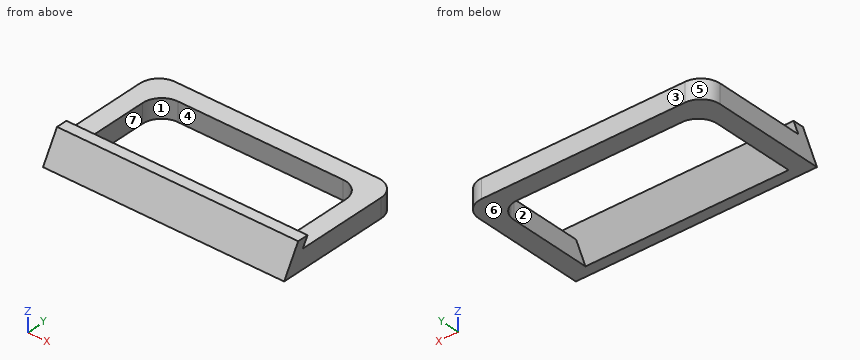
```python
from build123d import *

# Parameters (mm, degrees)
SALIENTE_EXTRUIR1_DEPTH = 10
SALIENTE_EXTRUIR2_DEPTH = 127


with BuildPart() as part:
    # Croquis1 → Saliente-Extruir1 (new body)
    with BuildSketch(Plane.XY):
        with BuildLine():
            Line((-36.931162, -5.25170068), (-36.931162, 48.74829932))
            ThreePointArc((-36.931162, 48.74829932), (-34.002229812, 55.819367132), (-26.931162, 58.74829932))
            Line((-26.931162, 58.74829932), (80.068838, 58.74829932))
            ThreePointArc((80.068838, 58.74829932), (87.139905812, 55.819367132), (90.068838, 48.74829932))
            Line((90.068838, 48.74829932), (90.068838, -5.25170068))
            Line((90.068838, -5.25170068), (80.068838, -5.25170068))
            Line((80.068838, -5.25170068), (80.068838, 38.74829932))
            ThreePointArc((80.068838, 38.74829932), (77.139905812, 45.819367132), (70.068838, 48.74829932))
            Line((70.068838, 48.74829932), (-16.931162, 48.74829932))
            ThreePointArc((-16.931162, 48.74829932), (-24.002229812, 45.819367132), (-26.931162, 38.74829932))
            Line((-26.931162, 38.74829932), (-26.931162, -5.25170068))
            Line((-26.931162, -5.25170068), (-36.931162, -5.25170068))
        make_face()
    extrude(amount=SALIENTE_EXTRUIR1_DEPTH)

    # Croquis2 → Saliente-Extruir2 (add)
    with BuildSketch(Plane.ZY.offset(36.931162)):
        Polygon((0, -11.025203372), (15, -2.364949334), (15, 3.408553358), (0, -5.25170068), align=None)
    extrude(amount=-SALIENTE_EXTRUIR2_DEPTH)


solid = part.part
```
For this review, take the finished solid that the model builds, in its own axes (mm). Face numbers are marked on the shaded views. A direction names the side the tool comes from. Coordinates: 2 decimals unless noted, no trailing zeros. Write each loop counter-clockwise with the first axis right and the second up, starting at its lowest first coordinate (ties: lowest second). Pieces come first, ordered by that corner, then holes. Notation, with made-up numbers: (76, -25.5) - (91, -25.5) arc R30 ccw to (91, -3.5) - close; hole circle Ø2 at (-28, 66.5). An arc over 180 degrees is marked (long way). Answer in a Markdown table with one row per item. Add a question column.
Q1. We need section A-A, the plane y = 28.5. State the section outline as (x, z) points, and give its area (3 significant figures).
Q2. We need section D-D, the plane y = 51.5. State the section outline as (x, z) points.
Q3. For probe 1 along X at (y, z) = (36, 2.75); probe 2 along Y at (x, z) = (43, 2.75); probe 3 along Z at (x, y) = (78, 48.5), list the stretches that pass through material, from the lowest coordinate up.
Q4. Tool access review of the marked faces 1, 2 and 3: name each direction out of +Z, -Z, +X, -X, +Y, -Y from which nothing blocks a thin tool from reaching the whole face with its end or side.
Q5. We need section B-B, the plane x = 65. State the section outline as (y, z) points.
Q6. We need section C-C, the plane z = 4.25. State the section outline as (x, y) points, and give its area (3 significant figures).
Q7. Draft analysis for pull direction Y (two halves, no side actions). For the marked faces 4, 5, 6 and 7, state which applies: +Y half, -Y half, draft (parallel to the pull), parting line (faces both ways), or undercut.
Q8. For P1, Ø1.5, axis at x = 52.5, z = 6.5, coming from the -Y side; P2, Ø1.5, axis at x = 7, z = 12, coming from the -Y side; P3, Ø6, axis at x = 59, y = -2.5, coming from the -Z side; P4, Ø8, axis at x = 62.5, z = 8.5, coming from the -Y side, all flat-tipped, find the tip position at first contact; note any pin that passes through.
Answer list:
| question | item | result |
|---|---|---|
| 1 | outline | (-36.93, 0) - (-26.93, 0) - (-26.93, 10) - (-36.93, 10) - close; (80.07, 0) - (90.07, 0) - (90.07, 10) - (80.07, 10) - close |
| 1 | area | 200 mm2 |
| 2 | outline | (-36.55, 0) - (89.68, 0) - (89.68, 10) - (-36.55, 10) - close |
| 3 | probe 1 | x = -36.93 to -26.93, 80.07 to 90.07 |
| 3 | probe 2 | y = -9.44 to -3.66, 48.75 to 58.75 |
| 3 | probe 3 | z = 0 to 10 |
| 4 | face 1 | +Z, -Z |
| 4 | face 2 | -Z |
| 4 | face 3 | +Z, -Z, +X, -X, +Y |
| 5 | outline | (-11.03, 0) - (-5.25, 0) - (3.41, 15) - (-2.36, 15) - close; (48.75, 0) - (58.75, 0) - (58.75, 10) - (48.75, 10) - close |
| 6 | outline | (-36.93, -8.57) - (90.07, -8.57) - (90.07, 48.75) arc R10 ccw to (80.07, 58.75) - (-26.93, 58.75) arc R10 ccw to (-36.93, 48.75) - close; hole (-26.93, -2.8) - (80.07, -2.8) - (80.07, 38.75) arc R10 ccw to (70.07, 48.75) - (-16.93, 48.75) arc R10 ccw to (-26.93, 38.75) - close |
| 6 | area | 3,030 mm2 |
| 7 | face 4 | undercut |
| 7 | face 5 | +Y half |
| 7 | face 6 | draft |
| 7 | face 7 | undercut |
| 8 | P1 | stops at y = -7.71 |
| 8 | P2 | stops at y = -4.53 |
| 8 | P3 | stops at z = 0 |
| 8 | P4 | stops at y = -8.43 |
